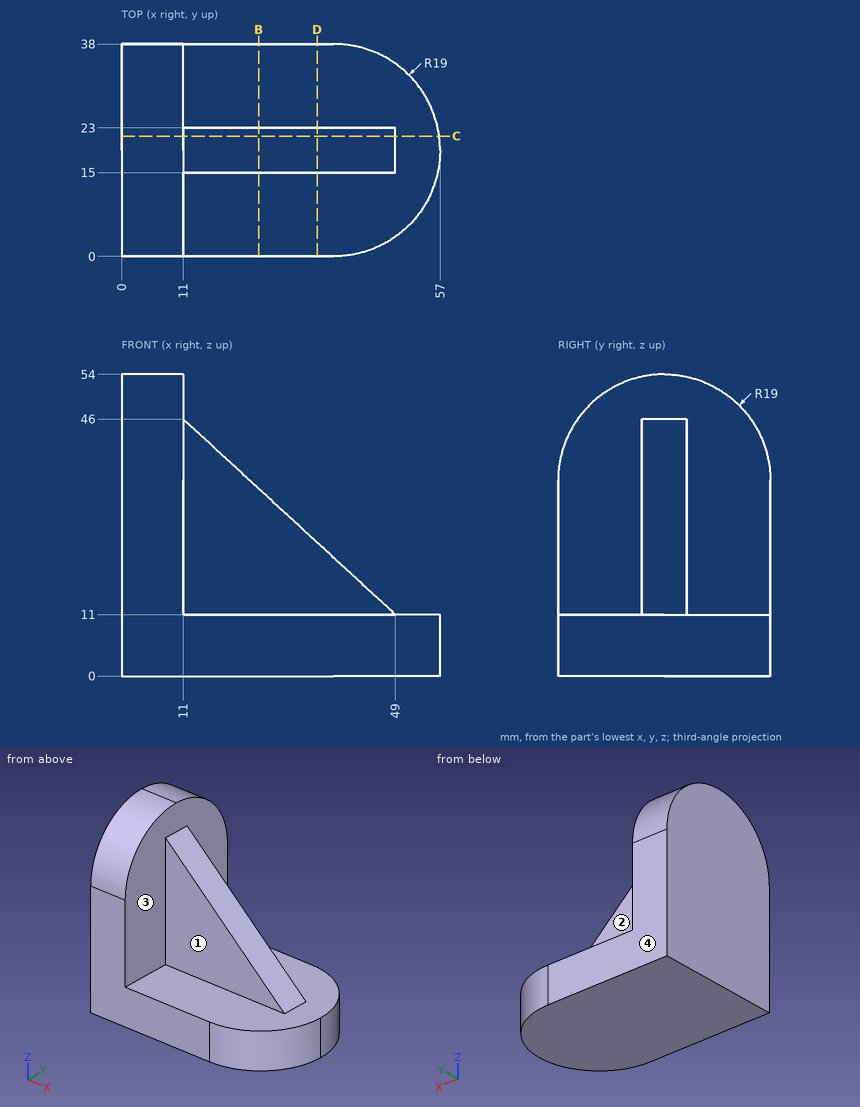
For this review, use the dimensioned drawing (mm, ordinates from the lowest corner) and the shaded views. A direction names the side the tool comes from. Round coordinates to 2 decimals unless told otherwise and drop trailing zeros. Order: outer loops, then holes, each group sorted by start corner. A loop starts at its lowest first (then second) coordinate and runs counter-clockwise, first axis right, second up.
1) Clearance check with flat-ended pins moving along their axes: pin 1 Ø17.5 at (x, z) = (21.5, 23.5) entering from -Y; pin 2 Ø12 at (y, z) = (13.5, 43.5) entering from +X; pin 3 Ø5 at (y, z) = (9.5, 44) entering from +X; pin 4 Ø4 at (y, z) = (27, 10) entering from -X. State where each tip first meets the part, or that it passes through.
The answers:
pin 1: stops at y = 15
pin 2: stops at x = 20.02
pin 3: stops at x = 11
pin 4: stops at x = 0
2) Machinability: for the marked faces 1, 2, 3 and 4, which of the approach directions +Z, -Z, +X, -X, +Y, -Y give a long, thin tool a straight path to every point of the face, cutting with its end or side? Answer none if there is none.
The answers:
face 1: +Z, +X, -Y
face 2: +Z, +X, +Y
face 3: +Z, +X, -Y
face 4: +Z, -Z, +X, -X, +Y
3) Consider section C-C (y = 21.5). State the section outline as (x, z) points.
The answers:
outline: (0, 0) - (56.83, 0) - (56.83, 11) - (49, 11) - (11, 46) - (11, 53.83) - (0, 53.83) - close
4) Consider section B-B (x = 24.5). State the section outline as (y, z) points, plus the area to 3 significant figures.
The answers:
outline: (0, 0) - (38, 0) - (38, 11) - (23, 11) - (23, 33.57) - (15, 33.57) - (15, 11) - (0, 11) - close
area: 599 mm2
5) For L1, parallel to Z at x = 21.5, y = 12.5; L2, parallel to Y at x = 36.5, z = 22, list the stretches that pass through material, from the lowest coordinate up.
The answers:
L1: z = 0 to 11
L2: y = 15 to 23
6) Consider section D-D (x = 35). State the section outline as (y, z) points, plus the area to 3 significant figures.
The answers:
outline: (0, 0) - (38, 0) - (38, 11) - (23, 11) - (23, 23.89) - (15, 23.89) - (15, 11) - (0, 11) - close
area: 521 mm2
